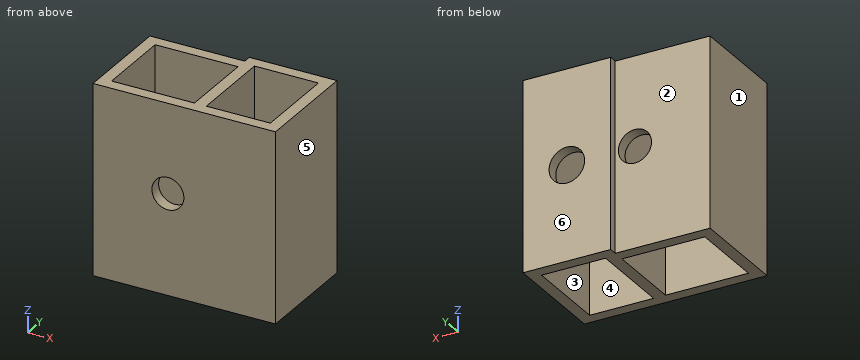
```python
from build123d import *

# Parameters (mm, degrees)
SKETCH1_W           = 44.45
SKETCH1_H           = 41.402
SKETCH1_W_2         = 34.29
SKETCH1_H_2         = 45.72
BOSS_EXTRUDE1_DEPTH = 101.6
SKETCH2_R           = 9.525
CUT_EXTRUDE1_DEPTH  = 12.7
SKETCH3_R           = 8.89
CUT_EXTRUDE2_DEPTH  = 12.7
SKETCH4_R           = 8.5725
CUT_EXTRUDE3_DEPTH  = 12.7


with BuildPart() as part:
    # Sketch1 → Boss-Extrude1 (new body)
    with BuildSketch(Plane.XY):
        Polygon((0, 0), (97.79, 0), (97.79, 58.42), (50.8, 58.42), (50.8, 54.102), (0, 54.102), align=None)
        with Locations((28.575, 27.051)):
            Rectangle(SKETCH1_W, SKETCH1_H, mode=Mode.SUBTRACT)
        with Locations((74.295, 29.21)):
            Rectangle(SKETCH1_W_2, SKETCH1_H_2, mode=Mode.SUBTRACT)
    extrude(amount=BOSS_EXTRUDE1_DEPTH)

    # Sketch2 → Cut-Extrude1 (cut)
    with BuildSketch(Plane(origin=(0, 58.42, 0), x_dir=(1, 0, 0), z_dir=(0, 1, 0))):
        with Locations(Location((74.295, -50.8, 0), (0, 0, 180))):
            Circle(SKETCH2_R)
    extrude(amount=-CUT_EXTRUDE1_DEPTH, mode=Mode.SUBTRACT)

    # Sketch3 → Cut-Extrude2 (cut)
    with BuildSketch(Plane(origin=(0, 54.102, 0), x_dir=(1, 0, 0), z_dir=(0, 1, 0))):
        with Locations(Location((40.240640863, -53.848, 0), (0, 0, 270))):
            Circle(SKETCH3_R)
    extrude(amount=-CUT_EXTRUDE2_DEPTH, mode=Mode.SUBTRACT)

    # Sketch4 → Cut-Extrude3 (cut)
    with BuildSketch(Plane(origin=(0, 6.35, 0), x_dir=(1, 0, 0), z_dir=(0, 1, 0))):
        with Locations(Location((40.132, -53.848, 0), (0, 0, 270))):
            Circle(SKETCH4_R)
    extrude(amount=-CUT_EXTRUDE3_DEPTH, mode=Mode.SUBTRACT)


solid = part.part
```
For this review, take the finished solid that the model builds, in its own axes (mm). Face numbers are marked on the shaded views. A direction names the side the tool comes from. Give positions to 0.01 mm unless a question says otherwise; leave off trailing zeros. Write each loop counter-clockwise with the first axis right and the second up, starting at its lowest first coordinate (ties: lowest second). Pieces come first, ordered by that corner, then holes. Notation, with made-up numbers: M 78,76 L 133,76 A20 ccw 133,92 Z; hole C 59.5,-22 d2. An arc over 180 degrees is marked long. One line per item, written item: value.
1) For P1, Ø13.5, axis at x = 32, z = 54.5, coming from the +Y side; P2, Ø2, axis at y = 56.5, z = 44, coming from the -X side, all flat-tipped, find the tip position at first contact; note any pin that passes through.
Results are:
P1: stops at y = 54.1
P2: stops at x = 50.8
2) The part is to be moulded in two halves that separate along X. For the marked faces 4, 5 and 6, say which applies: +X half, -X half, draft (parallel to the pull), parting line (faces both ways), or undercut.
Results are:
face 4: undercut
face 5: +X half
face 6: draft
3) For line 1 (X direction, y = 17, z = 90.5); line 2 (Y direction, x = 37.5, z = 19); line 3 (X direction, y = 53.5, z = 54.5), list the stretches that pass through material, from the lowest coordinate up. Write a range as from..to.
Results are:
line 1: x = 0..6.35, 50.8..57.15, 91.44..97.79
line 2: y = 0..6.35, 47.75..54.1
line 3: x = 0..31.37, 49.11..65.52, 83.07..97.79
4) Take a section at C-C, the plane z = 87. Write out the cut boundary in (x, y), then the cut area to 3 significant figures.
Results are:
outline: M 0,0 L 97.79,0 L 97.79,58.42 L 50.8,58.42 L 50.8,54.1 L 0,54.1 Z; hole M 6.35,6.35 L 50.8,6.35 L 50.8,47.75 L 6.35,47.75 Z; hole M 57.15,6.35 L 91.44,6.35 L 91.44,52.07 L 57.15,52.07 Z
area: 2,090 mm²
5) Take a section at D-D, the plane x = 69. Write out the cut boundary in (y, z).
Results are:
outline: M 0,0 L 6.35,0 L 6.35,101.6 L 0,101.6 Z; M 52.07,0 L 58.42,0 L 58.42,42.88 L 52.07,42.88 Z; M 52.07,58.72 L 58.42,58.72 L 58.42,101.6 L 52.07,101.6 Z
6) Take a section at A-A, the plane y = 12. Write out the cut boundary in (x, z).
Results are:
outline: M 0,0 L 6.35,0 L 6.35,101.6 L 0,101.6 Z; M 50.8,0 L 57.15,0 L 57.15,101.6 L 50.8,101.6 Z; M 91.44,0 L 97.79,0 L 97.79,101.6 L 91.44,101.6 Z
7) For the marked faces 1, 2 and 3, list the 3-axis set-ups (+Z, -Z, +X, -X, +Y, -Y) from which the entire face can be reached by the end or side of a thin tool; tool diameter is ignored.
Results are:
face 1: +Z, -Z, -X, +Y, -Y
face 2: +Z, -Z, -X, +Y
face 3: +Z, -Z
8) Take a section at B-B, the plane x = 87. Write out the cut boundary in (y, z).
Results are:
outline: M 0,0 L 6.35,0 L 6.35,101.6 L 0,101.6 Z; M 52.07,0 L 58.42,0 L 58.42,101.6 L 52.07,101.6 Z
